```python
from build123d import *

# Parameters (mm, degrees)
SKETCH1_R           = 7
BOSS_EXTRUDE1_DEPTH = 1.8
SKETCH2_R           = 0.75
CUT_EXTRUDE1_DEPTH  = 11.061808982
CIRPATTERN1_COUNT   = 6


with BuildPart() as part:
    # Sketch1 → Boss-Extrude1 (new body)
    with BuildSketch(Plane(origin=(0, 0, 0), x_dir=(1, 0, 0), z_dir=(0, 1, 0))):
        with Locations(Location((0, 0, 0), (0, 0, 270))):
            Circle(SKETCH1_R)
    extrude(amount=BOSS_EXTRUDE1_DEPTH)

    # Sketch2 → Cut-Extrude1 (cut, through all)
    with BuildSketch(Plane.XZ):
        with Locations(Location((0, 5.873718021, 0), (0, 0, 270))):
            Circle(SKETCH2_R)
    cut_extrude1 = extrude(amount=-CUT_EXTRUDE1_DEPTH, mode=Mode.SUBTRACT)

    # CirPattern1: Cut-Extrude1 ×6 about axis
    cirpattern1_axis = Axis((0, 0, 0), (0, 1, 0))
    for i in range(1, CIRPATTERN1_COUNT):
        add(cut_extrude1.rotate(cirpattern1_axis, i * 360 / CIRPATTERN1_COUNT), mode=Mode.SUBTRACT)


solid = part.part
```
Geometry check sheet. Reference: the model listing, model coordinates, mm. Give positions to 0.01 mm unless a question says otherwise; leave off trailing zeros. Order: outer loops, then holes, each group sorted by start corner. A loop starts at its lowest first (then second) coordinate and runs counter-clockwise, first axis right, second up. Notation, with made-up numbers: (-19.5, 11.5) -> (33.5, 11.5) arc R21 ccw to (33.5, 34.5) -> close; hole circle Ø2 at (69, -39.75). An arc over 180 degrees is marked (long way). Write each question's results on one line, items separated by ' | '. Start each with the question number.
(1) Sectioned sample at A-A (x = 0). Enter the section's corners in (y, z).
(2) Sectioned sample at D-D (x = 3). Enter the section's corners in (y, z).
(3) Scan lines: line 1 (X direction, y = 1.6, z = 3); line 2 (Z direction, x = 0.25, y = 0.8); line 3 (X direction, y = 0.2, z = 3.25). Record each from-to range of solid material in increasing order.
(4) Sectioned sample at B-B (z = -3). Enter the section's corners in (x, y).
(5) Mould release check, pull along Z, two halves, no side actions. Record for faces 1 (the face through (-0.033, 0.887, -6.623)), 2 (the face through (0, 1.8, 0)), 3 (the face through (-6.834, 0.887, -1.517)): pulls with the +Z half, pulls with the -Z half, needs draft (parallel to the pull), parting line crosses it, or undercut.
(6) Sectioned sample at C-C (y = 1.6). Enter the section's corners in (x, z).
Answer below:
1) outline: (0, -7) -> (1.8, -7) -> (1.8, -6.62) -> (0, -6.62) -> close; (0, -5.12) -> (1.8, -5.12) -> (1.8, 5.12) -> (0, 5.12) -> close; (0, 6.62) -> (1.8, 6.62) -> (1.8, 7) -> (0, 7) -> close
2) outline: (0, -6.32) -> (1.8, -6.32) -> (1.8, 6.32) -> (0, 6.32) -> close
3) line 1: -6.32 to -5.83, -4.34 to 4.34, 5.83 to 6.32 | line 2: -7 to -6.58, -5.17 to 5.17, 6.58 to 7 | line 3: -6.2 to -5.77, -4.41 to 4.41, 5.77 to 6.2
4) outline: (-6.32, 0) -> (-5.83, 0) -> (-5.83, 1.8) -> (-6.32, 1.8) -> close; (-4.34, 0) -> (4.34, 0) -> (4.34, 1.8) -> (-4.34, 1.8) -> close; (5.83, 0) -> (6.32, 0) -> (6.32, 1.8) -> (5.83, 1.8) -> close
5) face 1: undercut | face 2: needs draft | face 3: parting line crosses it
6) outline: circle Ø14 at (0, 0); hole circle Ø1.5 at (-5.09, -2.94); hole circle Ø1.5 at (-5.09, 2.94); hole circle Ø1.5 at (0, -5.87); hole circle Ø1.5 at (0, 5.87); hole circle Ø1.5 at (5.09, -2.94); hole circle Ø1.5 at (5.09, 2.94)
